Part model, mm, in its own coordinate system. A direction names the side the tool comes from. Coordinates: 2 decimals unless noted, no trailing zeros. Write each loop counter-clockwise with the first axis right and the second up, starting at its lowest first coordinate (ties: lowest second). Pieces come first, ordered by that corner, then holes. Notation, with made-up numbers: (35.25, 89) - (60.25, 89) arc R27 ccw to (60.25, 112) - close; hole circle Ø8 at (-2, 6.25). An arc over 180 degrees is marked (long way). Use a Markdown table: item, result.
```python
from build123d import *

# Parameters (mm, degrees)
SKETCH1_W             = 1
SKETCH1_H             = 8
REVOLVE1_ANGLE        = 180
SKETCH2_R             = 1.6
BOSS_EXTRUDE1_DEPTH   = 2
BOSS_EXTRUDE1_2_DEPTH = 2
REVOLVE2_ANGLE        = 180


with BuildPart() as part:
    # Sketch1 → Revolve1 (revolve)
    with BuildSketch(Plane.XY):
        Polygon((-1.8, -3), (-1.8, 0), (-2.8, 0), (-7.8, 0), (-10.8, 0), (-10.8, -3), align=None)
        Polygon((-10.8, 0), (-3.8, 8), (-7.8, 0), align=None)
        with Locations((-2.3, 4)):
            Rectangle(SKETCH1_W, SKETCH1_H)
    revolve(axis=Axis((0, 0, 0), (0, 1, 0)), revolution_arc=REVOLVE1_ANGLE)



with BuildPart() as body_2:
    # Sketch2 → Boss-Extrude1 (new body)
    with BuildSketch(Plane(origin=(0, 0, 0), x_dir=(-1, 0, 0), z_dir=(0, 0, -1))):
        Polygon((-10.8, -3), (-16.8, -3), (-16.8, 2.254410697), (-11.77260936, 8), (-3.8, 8), (-10.8, 0), align=None)
        with Locations((-10.41130468, 5)):
            Circle(SKETCH2_R, mode=Mode.SUBTRACT)
        with Locations((-13.8, 0)):
            Circle(SKETCH2_R, mode=Mode.SUBTRACT)
    extrude(amount=-BOSS_EXTRUDE1_DEPTH)


with BuildPart() as body_3:
    # Sketch2 → Boss-Extrude1 2 (new body)
    with BuildSketch(Plane(origin=(0, 0, 0), x_dir=(-1, 0, 0), z_dir=(0, 0, -1))):
        Polygon((10.8, 0), (3.8, 8), (11.77260936, 8), (16.8, 2.254410697), (16.8, -3), (10.8, -3), align=None)
        with Locations(Location((13.8, 0, 0), (0, 0, 180))):
            Circle(SKETCH2_R, mode=Mode.SUBTRACT)
        with Locations(Location((10.41130468, 5, 0), (0, 0, 180))):
            Circle(SKETCH2_R, mode=Mode.SUBTRACT)
    extrude(amount=-BOSS_EXTRUDE1_2_DEPTH)


with BuildPart() as part_1:
    add(part.part)

    add(body_2.part)  # Revolve2 merges body 2

    add(body_3.part)  # Revolve2 merges body 3
    # Sketch3 → Revolve2 (revolve)
    with BuildSketch(Plane(origin=(0, 0, 0), x_dir=(-1, 0, 0), z_dir=(0, 0, -1))):
        Polygon((-11.8, -3), (-11.8, 0), (-4.8, 8), (-3.8, 8), (-10.8, 0), (-10.8, -3), align=None)
    revolve(axis=Axis((0, 0, 0), (0, -1, 0)), revolution_arc=REVOLVE2_ANGLE)


solid = part_1.part
```
Item 1: Band-saw the part on A-A, the plane y = -2. Give the cut face in (x, z), then the cut area to 3 significant figures.
From the geometry:
| item | result |
|---|---|
| outline | (-16.8, 0) - (-1.8, 0) arc R1.8 cw to (1.8, 0) - (16.8, 0) - (16.8, 2) - (11.63, 2) arc R11.8 ccw to (-11.63, 2) - (-16.8, 2) - close |
| area | 234 mm^2 |
Item 2: Which spindle directions (+Z, -Z, +X, -X, +Y, -Y) get a long thin tool onto all of the face, cutting with end or side? Do faces 5 (the face through (-12, 3, 2)), 6 (the face through (-0.1, 4.1, 2.8)), 7 (the face through (-0.1, 4.8, 5.4)). Say none if no direction does.
From the geometry:
| item | result |
|---|---|
| face 5 | +Z, -X, +Y |
| face 6 | +Y |
| face 7 | none |
Item 3: Two-plate mould, pull along X, no slides. Class faces 1 (the face through (0, 2.6, 1.8)), 2 (the face through (12, 4, 2)), 3 (the face through (0, 0, 4)), 4 (the face through (0.2, -1.5, 11.8)): pulls with the +X half, pulls with the -X half, needs draft (parallel to the pull), parting line crosses it, or undercut.
From the geometry:
| item | result |
|---|---|
| face 1 | undercut |
| face 2 | needs draft |
| face 3 | undercut |
| face 4 | parting line crosses it |
Item 4: Band-saw the part on D-D, the plane y = 6.25. Count the separate pieces of the cut face and the enclosed holes in it, then the cut area to 3 significant figures.
From the geometry:
| item | result |
|---|---|
| separate pieces | 4 |
| enclosed holes | 0 |
| area | 56.2 mm^2 |
Item 5: Drill centre lines: probe 1 along X at (y, z) = (-2, 1.5); probe 2 along Z at (x, y) = (-13.5, 4.5); probe 3 along Y at (x, z) = (-4, 2.75). Where is each one in solid material? Low to high.
From the geometry:
| item | result |
|---|---|
| probe 1 | -16.8 to -0.99, 0.99 to 16.8 |
| probe 2 | 0 to 2 |
| probe 3 | -3 to 0, 5.89 to 7.94 |
Item 6: Band-saw the part on B-B, the plane x = 13.8. Give the cut face in (y, z), then the cut area to 3 significant figures.
From the geometry:
| item | result |
|---|---|
| outline | (-3, 0) - (-1.6, 0) - (-1.6, 2) - (-3, 2) - close; (1.6, 0) - (5.68, 0) - (5.68, 2) - (1.6, 2) - close |
| area | 11.0 mm^2 |
Item 7: Band-saw the part on C-C, the plane y = 3. Give the cut face in (x, z) (3 decimals), then the cut area to 3 significant figures.
From the geometry:
| item | result |
|---|---|
| outline | (-16.148, 0) - (-6.3, 0) arc R6.3 cw to (6.3, 0) - (16.148, 0) - (16.148, 2) - (8.954, 2) arc R9.175 ccw to (-8.954, 2) - (-16.148, 2) - close; (-2.8, 0) - (-1.8, 0) arc R1.8 cw to (1.8, 0) - (2.8, 0) arc R2.8 ccw to start |
| area | 105 mm^2 |
Item 8: Drop flat-ended pins along their axis: P1, Ø6, axis at y = 5, z = 9, coming from the +X side; P2, Ø3, axis at x = -10.41, y = 5, coming from the -Z side; P3, Ø6, axis at x = 12.5, y = 6, coming from the +Z side; P4, Ø1, axis at x = 1, y = 2, coming from the -Z side (3 decimals). Give the stop position or say it passes through.
From the geometry:
| item | result |
|---|---|
| P1 | x = 6.25 |
| P2 | through |
| P3 | z = 2 |
| P4 | z = 0.995 |
